Design review of the part built by this model. Coordinates are the model's own, in mm. A direction names the side the tool comes from. Coordinates: 2 decimals unless noted, no trailing zeros. Order: outer loops, then holes, each group sorted by start corner. A loop starts at its lowest first (then second) coordinate and runs counter-clockwise, first axis right, second up. Notation, with made-up numbers: M 31,18.5 L 63,18.5 A19 cw 63,53.5 Z; hole C -14.5,31.5 d10. An arc over 180 degrees is marked long. Answer in a Markdown table with one row per item.
from build123d import *

# Parameters (mm, degrees)
SKETCH2_R                            = 2.0193
BOSS_EXTRUDE1_DEPTH                  = 307.975
SKETCH7_R                            = 6.35
BOSS_EXTRUDE2_DEPTH                  = 7.9375
F_10_32_TAPPED_HOLE2_D               = 4.0386
F_10_32_TAPPED_HOLE2_DEPTH           = 16.34744
F_10_32_TAPPED_HOLE2_TIP             = 1.213317848
F_10_32_TAPPED_HOLE2_ON_FACE_2_D     = 4.0386
F_10_32_TAPPED_HOLE2_ON_FACE_2_DEPTH = 16.34744
F_10_32_TAPPED_HOLE2_ON_FACE_2_TIP   = 1.213317848


with BuildPart() as part:
    # Sketch2 → Boss-Extrude1 (new, symmetric)
    with BuildSketch(Plane.XY):
        with BuildLine():
            ThreePointArc((0.93173274, 6.79441227), (0, 6.858), (-0.93173274, 6.79441227))
            Line((-0.93173274, 6.79441227), (-5.41826726, 4.204110358))
            ThreePointArc((-5.41826726, 4.204110358), (-5.939202219, 3.429), (-6.35, 2.590301913))
            Line((-6.35, 2.590301913), (-6.35, -2.590301913))
            ThreePointArc((-6.35, -2.590301913), (-5.939202219, -3.429), (-5.41826726, -4.204110358))
            Line((-5.41826726, -4.204110358), (-0.93173274, -6.79441227))
            ThreePointArc((-0.93173274, -6.79441227), (0, -6.858), (0.93173274, -6.79441227))
            Line((0.93173274, -6.79441227), (5.41826726, -4.204110358))
            ThreePointArc((5.41826726, -4.204110358), (5.939202219, -3.429), (6.35, -2.590301913))
            Line((6.35, -2.590301913), (6.35, 2.590301913))
            ThreePointArc((6.35, 2.590301913), (5.939202219, 3.429), (5.41826726, 4.204110358))
            Line((5.41826726, 4.204110358), (0.93173274, 6.79441227))
        make_face()
        Circle(SKETCH2_R, mode=Mode.SUBTRACT)
    extrude(amount=BOSS_EXTRUDE1_DEPTH, both=True)

    # Sketch7 → Boss-Extrude2 (add)
    with BuildSketch(Plane.XY.offset(307.975)):
        Circle(SKETCH7_R)
    boss_extrude2 = extrude(amount=BOSS_EXTRUDE2_DEPTH)

    # Mirror1: Boss-Extrude2 across plane
    add(boss_extrude2.mirror(Plane.XY))

    # #10-32 Tapped Hole2
    with Locations(Plane.XY.offset(315.9125)):
        with Locations((0, 0)):
            Hole(F_10_32_TAPPED_HOLE2_D / 2, depth=F_10_32_TAPPED_HOLE2_DEPTH)
            with Locations((0, 0, -(F_10_32_TAPPED_HOLE2_DEPTH + F_10_32_TAPPED_HOLE2_TIP / 2))):  # 118° drill point
                Cone(0, F_10_32_TAPPED_HOLE2_D / 2, F_10_32_TAPPED_HOLE2_TIP, mode=Mode.SUBTRACT)

    # #10-32 Tapped Hole2 on face 2
    with Locations(Plane(origin=(0, 0, -315.9125), x_dir=(-1, 0, 0), z_dir=(0, 0, -1))):
        with Locations((0, 0)):
            Hole(F_10_32_TAPPED_HOLE2_ON_FACE_2_D / 2, depth=F_10_32_TAPPED_HOLE2_ON_FACE_2_DEPTH)
            with Locations((0, 0, -(F_10_32_TAPPED_HOLE2_ON_FACE_2_DEPTH + F_10_32_TAPPED_HOLE2_ON_FACE_2_TIP / 2))):  # 118° drill point
                Cone(0, F_10_32_TAPPED_HOLE2_ON_FACE_2_D / 2, F_10_32_TAPPED_HOLE2_ON_FACE_2_TIP, mode=Mode.SUBTRACT)


solid = part.part
(1) For faces 1 (the cylindrical face through (-1.38, -6.2, -311.89)), 2 (the cylindrical face through (-1.38, -6.2, 311.89)), 3 (the flat face through (-2, 2, -315.912)), list the 3-axis set-ups (+Z, -Z, +X, -X, +Y, -Y) from which the entire face can be reached by the end or side of a thin tool; tool diameter is ignored.
Return value:
| item | result |
|---|---|
| face 1 | -Z |
| face 2 | +Z |
| face 3 | -Z, +X, -X, +Y, -Y |
(2) For line 1 along Y through (x, z) = (0, 149.5); line 2 along X through (y, z) = (0, 313.5), list the stretches that pass through material, from the lowest coordinate up. Write a range as from..to.
Return value:
| item | result |
|---|---|
| line 1 | y = -6.86..-2.02, 2.02..6.86 |
| line 2 | x = -6.35..-2.02, 2.02..6.35 |
(3) Add section A-A, the plane z = -231. Give the boundary of the cut face in (x, y), and give its area (3 significant figures).
Return value:
| item | result |
|---|---|
| outline | M -6.35,-2.59 A6.86 ccw -5.42,-4.2 L -0.93,-6.79 A6.86 ccw 0.93,-6.79 L 5.42,-4.2 A6.86 ccw 6.35,-2.59 L 6.35,2.59 A6.86 ccw 5.42,4.2 L 0.93,6.79 A6.86 ccw -0.93,6.79 L -5.42,4.2 A6.86 ccw -6.35,2.59 Z; hole C 0,0 d4.04 |
| area | 124 mm2 |
(4) Insertion check: pin 1 Ø3.5 at (x, y) = (-5, -4) entering from +Z. The pin has a flat end and moves straight along its axis. Give the tip position at first contact, or say it passes through.
Return value:
| item | result |
|---|---|
| pin 1 | stops at z = 315.91 |
